from build123d import *

# Parameters (mm, degrees)
SKETCH2_W           = 15
SKETCH2_H           = 8
SKETCH2_W_2         = 30
SKETCH2_W_3         = 7.5
SKETCH2_H_2         = 10
BOSS_EXTRUDE1_DEPTH = 2
SKETCH3_W           = 52.5
SKETCH3_H           = 30
BOSS_EXTRUDE2_DEPTH = 2


with BuildPart() as part:
    # Sketch2 → Boss-Extrude1 (new body)
    with BuildSketch(Plane.XY):
        with Locations((-15, 90)):
            Rectangle(SKETCH2_W, SKETCH2_H)
        with Locations((7.5, 90)):
            Rectangle(SKETCH2_W_2, SKETCH2_H)
        with Locations((26.25, 90)):
            Rectangle(SKETCH2_W_3, SKETCH2_H)
        with Locations((26.25, 81)):
            Rectangle(SKETCH2_W_3, SKETCH2_H_2)
        with Locations((26.25, 72)):
            Rectangle(SKETCH2_W_3, SKETCH2_H)
        with Locations((7.5, 72)):
            Rectangle(SKETCH2_W_2, SKETCH2_H)
        with Locations((-15, 72)):
            Rectangle(SKETCH2_W, SKETCH2_H)
        with Locations((-15, 81)):
            Rectangle(SKETCH2_W, SKETCH2_H_2)
        with Locations((-15, 63)):
            Rectangle(SKETCH2_W, SKETCH2_H_2)
        with Locations((-15, 54)):
            Rectangle(SKETCH2_W, SKETCH2_H)
        with Locations((7.5, 54)):
            Rectangle(SKETCH2_W_2, SKETCH2_H)
        with Locations((26.25, 54)):
            Rectangle(SKETCH2_W_3, SKETCH2_H)
        with Locations((26.25, 63)):
            Rectangle(SKETCH2_W_3, SKETCH2_H_2)
        with Locations((-15, 45)):
            Rectangle(SKETCH2_W, SKETCH2_H_2)
        with Locations((-15, 36)):
            Rectangle(SKETCH2_W, SKETCH2_H)
        with Locations((-15, 27)):
            Rectangle(SKETCH2_W, SKETCH2_H_2)
        with Locations((-15, -90)):
            Rectangle(SKETCH2_W, SKETCH2_H)
        with Locations((7.5, -90)):
            Rectangle(SKETCH2_W_2, SKETCH2_H)
        with Locations((26.25, -90)):
            Rectangle(SKETCH2_W_3, SKETCH2_H)
        with Locations((26.25, -81)):
            Rectangle(SKETCH2_W_3, SKETCH2_H_2)
        with Locations((-15, -81)):
            Rectangle(SKETCH2_W, SKETCH2_H_2)
        with Locations((-15, -72)):
            Rectangle(SKETCH2_W, SKETCH2_H)
        with Locations((7.5, -72)):
            Rectangle(SKETCH2_W_2, SKETCH2_H)
        with Locations((26.25, -72)):
            Rectangle(SKETCH2_W_3, SKETCH2_H)
        with Locations((26.25, -63)):
            Rectangle(SKETCH2_W_3, SKETCH2_H_2)
        with Locations((26.25, -54)):
            Rectangle(SKETCH2_W_3, SKETCH2_H)
        with Locations((7.5, -54)):
            Rectangle(SKETCH2_W_2, SKETCH2_H)
        with Locations((-15, -54)):
            Rectangle(SKETCH2_W, SKETCH2_H)
        with Locations((-15, -63)):
            Rectangle(SKETCH2_W, SKETCH2_H_2)
        with Locations((-15, -45)):
            Rectangle(SKETCH2_W, SKETCH2_H_2)
        with Locations((-15, -36)):
            Rectangle(SKETCH2_W, SKETCH2_H)
        with Locations((-15, -27)):
            Rectangle(SKETCH2_W, SKETCH2_H_2)
        with Locations((-15, -18)):
            Rectangle(SKETCH2_W, SKETCH2_H)
        with Locations((-15, -9)):
            Rectangle(SKETCH2_W, SKETCH2_H_2)
        with Locations((7.5, -36)):
            Rectangle(SKETCH2_W_2, SKETCH2_H)
        with Locations((26.25, -36)):
            Rectangle(SKETCH2_W_3, SKETCH2_H)
        with Locations((26.25, -45)):
            Rectangle(SKETCH2_W_3, SKETCH2_H_2)
        with Locations((26.25, -27)):
            Rectangle(SKETCH2_W_3, SKETCH2_H_2)
        with Locations((26.25, -18)):
            Rectangle(SKETCH2_W_3, SKETCH2_H)
        with Locations((7.5, -18)):
            Rectangle(SKETCH2_W_2, SKETCH2_H)
        with Locations((26.25, -9)):
            Rectangle(SKETCH2_W_3, SKETCH2_H_2)
        with Locations((-15, 0)):
            Rectangle(SKETCH2_W, SKETCH2_H)
        with Locations((7.5, 0)):
            Rectangle(SKETCH2_W_2, SKETCH2_H)
        with Locations((26.25, 0)):
            Rectangle(SKETCH2_W_3, SKETCH2_H)
        with Locations((26.25, 9)):
            Rectangle(SKETCH2_W_3, SKETCH2_H_2)
        with Locations((-15, 9)):
            Rectangle(SKETCH2_W, SKETCH2_H_2)
        with Locations((-15, 18)):
            Rectangle(SKETCH2_W, SKETCH2_H)
        with Locations((7.5, 36)):
            Rectangle(SKETCH2_W_2, SKETCH2_H)
        with Locations((7.5, 18)):
            Rectangle(SKETCH2_W_2, SKETCH2_H)
        with Locations((26.25, 18)):
            Rectangle(SKETCH2_W_3, SKETCH2_H)
        with Locations((26.25, 27)):
            Rectangle(SKETCH2_W_3, SKETCH2_H_2)
        with Locations((26.25, 36)):
            Rectangle(SKETCH2_W_3, SKETCH2_H)
        with Locations((26.25, 45)):
            Rectangle(SKETCH2_W_3, SKETCH2_H_2)
    extrude(amount=BOSS_EXTRUDE1_DEPTH)

    # Sketch3 → Boss-Extrude2 (add)
    with BuildSketch(Plane.XY.offset(2)):
        with Locations((3.75, -109)):
            Rectangle(SKETCH3_W, SKETCH3_H)
    extrude(amount=-BOSS_EXTRUDE2_DEPTH)


solid = part.part
Geometry check sheet. Reference: the model listing, model coordinates, mm. Give positions to 0.01 mm unless a question says otherwise; leave off trailing zeros. Write each loop counter-clockwise with the first axis right and the second up, starting at its lowest first coordinate (ties: lowest second). Pieces come first, ordered by that corner, then holes. Notation, with made-up numbers: (-15, -20.75) - (-8, -20.75) arc R22 cw to (-8, 15.25) - close; hole circle Ø5 at (-27, 60.25). An arc over 180 degrees is marked (long way). Put each result on its own line as item: value.
1. Sectioned sample at B-B, the plane x = 16.5. Give the number of separate pieces and of enclosed holes in the cut face, plus the area to 3 significant figures.
Ans:
separate pieces: 11
enclosed holes: 0
area: 236 mm²
2. Thickness scan on line 1 (X direction, y = -59.5, z = 0.65). Record the ranges inside material, lowest first.
Ans:
line 1: x = -22.5 to -7.5, 22.5 to 30
3. Sectioned sample at A-A, the plane y = -9.5. Enter the section's corners in (x, z), plus the area to 3 significant figures.
Ans:
outline: (-22.5, 0) - (-7.5, 0) - (-7.5, 2) - (-22.5, 2) - close; (22.5, 0) - (30, 0) - (30, 2) - (22.5, 2) - close
area: 45.0 mm²
